Verification items for the finished model (mm, model axes). A direction names the side the tool comes from. Round coordinates to 2 decimals unless told otherwise and drop trailing zeros. Write each loop counter-clockwise with the first axis right and the second up, starting at its lowest first coordinate (ties: lowest second). Pieces come first, ordered by that corner, then holes. Notation, with made-up numbers: (59, -20) -> (111, -20) arc R4 ccw to (111, -16) -> close; hole circle Ø2 at (66, -38). An arc over 180 degrees is marked (long way). Use CSV: the item, a comma, the result in double quotes.
```python
from build123d import *

# Parameters (mm, degrees)
BOSS_EXTRUDE1_DEPTH                                = 304.8
SKETCH2_R                                          = 2.3876
CUT_EXTRUDE1_DEPTH                                 = 317.354227758
SKETCH3_R                                          = 11.1125
CUT_EXTRUDE2_DEPTH                                 = 304.8
CSK_FOR_10_FLAT_HEAD_MACHINE_SCREW1_AT_COUNT       = 2
CSK_FOR_10_FLAT_HEAD_MACHINE_SCREW1_AT_PITCH       = 41.275
LPATTERN1_COUNT                                    = 2
LPATTERN1_PITCH                                    = 171.958
FILLET1_R                                          = 6.35
SKETCH14_R                                         = 4.8895
SKETCH14_R_2                                       = 2.8067
BOSS_EXTRUDE2_DEPTH                                = 3.175
CONVERT_SOLID1_DEPTH                               = 304.8
F_10_0_1935_DIAMETER_HOLE1_D                       = 4.9149
F_10_0_1935_DIAMETER_HOLE1_DEPTH                   = 3.048
CSK_FOR_10_FLAT_HEAD_MACHINE_SCREW_100_D           = 5.6134
CSK_FOR_10_FLAT_HEAD_MACHINE_SCREW_100_DEPTH       = 36.8935
CSK_FOR_10_FLAT_HEAD_MACHINE_SCREW_100_CSINK_D     = 9.779
CSK_FOR_10_FLAT_HEAD_MACHINE_SCREW_100_CSINK_ANGLE = 82


# Read off the part's stored shape, not the designer's step: Convert-Solid1
with BuildPart() as part:
    # Sketch1 → Boss-Extrude1 (new body)
    with BuildSketch(Plane(origin=(0, 0, 0), x_dir=(0, 0, -1), z_dir=(1, 0, 0))):
        with BuildLine():
            Line((-76.2, 4.2545), (-53.975, 4.2545))
            ThreePointArc((-53.975, 4.2545), (-49.484871939, 6.114371939), (-47.625, 10.6045))
            Line((-47.625, 10.6045), (-47.625, 34.925))
            ThreePointArc((-47.625, 34.925), (-46.69506403, 37.17006403), (-44.45, 38.1))
            Line((-44.45, 38.1), (44.45, 38.1))
            ThreePointArc((44.45, 38.1), (46.69506403, 37.17006403), (47.625, 34.925))
            Line((47.625, 34.925), (47.625, 10.6045))
            ThreePointArc((47.625, 10.6045), (49.484871939, 6.114371939), (53.975, 4.2545))
            Line((53.975, 4.2545), (76.2, 4.2545))
            Line((76.2, 4.2545), (76.2, 7.4295))
            Line((76.2, 7.4295), (53.975, 7.4295))
            ThreePointArc((53.975, 7.4295), (51.72993597, 8.35943597), (50.8, 10.6045))
            Line((50.8, 10.6045), (50.8, 34.925))
            ThreePointArc((50.8, 34.925), (48.940128061, 39.415128061), (44.45, 41.275))
            Line((44.45, 41.275), (-44.45, 41.275))
            ThreePointArc((-44.45, 41.275), (-48.940128061, 39.415128061), (-50.8, 34.925))
            Line((-50.8, 34.925), (-50.8, 10.6045))
            ThreePointArc((-50.8, 10.6045), (-51.72993597, 8.35943597), (-53.975, 7.4295))
            Line((-53.975, 7.4295), (-76.2, 7.4295))
            Line((-76.2, 7.4295), (-76.2, 4.2545))
        make_face()
    extrude(amount=BOSS_EXTRUDE1_DEPTH)

    # Sketch2 → Cut-Extrude1 (cut, through all)
    with BuildSketch(Plane.XZ.offset(-4.2545)):
        with Locations(Location((25.4, 63.5, 0), (0, 0, 270))):
            Circle(SKETCH2_R)
        with Locations(Location((152.4, 63.5, 0), (0, 0, 270))):
            Circle(SKETCH2_R)
        with Locations(Location((279.4, 63.5, 0), (0, 0, 270))):
            Circle(SKETCH2_R)
    cut_extrude1 = extrude(amount=-CUT_EXTRUDE1_DEPTH, mode=Mode.SUBTRACT)

    # Mirror1: Cut-Extrude1 across plane
    add(cut_extrude1.mirror(Plane.XY), mode=Mode.SUBTRACT)

    # Sketch3 → Cut-Extrude2 (cut)
    with BuildSketch(Plane(origin=(0, 41.275, 0), x_dir=(1, 0, 0), z_dir=(0, 1, 0))):
        with Locations(Location((66.675, -15.875, 0), (0, 0, 270))):
            Circle(SKETCH3_R)
    cut_extrude2 = extrude(amount=-CUT_EXTRUDE2_DEPTH, mode=Mode.SUBTRACT)

    # Sketch5 → CSK for #10 Flat Head Machine Screw1 (revolve, cut)
    with BuildSketch(Plane(origin=(46.0375, 41.275, 15.875), x_dir=(0, 0, 1), z_dir=(1, 0, 0))):
        Polygon((0, 0), (0, 3.175), (2.8067, 3.175), (2.8067, 2.395987319), (4.8895, 0), align=None)
    csk_for_10_flat_head_machine_screw1 = revolve(axis=Axis((46.0375, 47.625, 15.875), (0, -1, 0)), mode=Mode.SUBTRACT)

    # CSK for #10 Flat Head Machine Screw1 at: CSK for #10 Flat Head Machine Screw1 ×2
    with Locations(*[(i * CSK_FOR_10_FLAT_HEAD_MACHINE_SCREW1_AT_PITCH, 0, 0) for i in range(1, CSK_FOR_10_FLAT_HEAD_MACHINE_SCREW1_AT_COUNT)]):
        add(csk_for_10_flat_head_machine_screw1, mode=Mode.SUBTRACT)

    # LPattern1: Cut-Extrude2, CSK for #10 Flat Head Machine Screw1 ×2
    with Locations(*[(i * LPATTERN1_PITCH, 0, 0) for i in range(1, LPATTERN1_COUNT)]):
        add(cut_extrude2, mode=Mode.SUBTRACT)
        add(csk_for_10_flat_head_machine_screw1, mode=Mode.SUBTRACT)

    # LPattern1 copy 1 sketch → LPattern1 copy 1 (revolve, cut)
    with BuildSketch(Plane(origin=(259.2705, 41.275, 15.875), x_dir=(0, 0, 1), z_dir=(1, 0, 0))):
        Polygon((0, 0), (0, 3.175), (2.8067, 3.175), (2.8067, 2.395987319), (4.8895, 0), align=None)
    revolve(axis=Axis((259.2705, 47.625, 15.875), (0, -1, 0)), mode=Mode.SUBTRACT)

    # Fillet1
    fillet1_edges = [part.edges().sort_by_distance(p)[0] for p in [
        (0, 5.842, -76.2),
        (0, 5.842, 76.2),
        (304.8, 5.842, -76.2),
        (304.8, 5.842, 76.2),
    ]]
    fillet(fillet1_edges, radius=FILLET1_R)

    # Sketch14 → Boss-Extrude2 (add)
    # profile 1 of 4: a face of its own
    with BuildSketch(Plane(origin=(0, 41.275, 0), x_dir=(1, 0, 0), z_dir=(0, 1, 0))):
        with Locations((259.2705, -15.875)):
            Circle(SKETCH14_R)
        with Locations(Location((259.2705, -15.875, 0), (0, 0, 270))):
            Circle(SKETCH14_R_2, mode=Mode.SUBTRACT)
    # profile 2 of 4: a face of its own
    with BuildSketch(Plane(origin=(0, 41.275, 0), x_dir=(1, 0, 0), z_dir=(0, 1, 0))):
        with Locations((87.3125, -15.875)):
            Circle(SKETCH14_R)
        with Locations(Location((87.3125, -15.875, 0), (0, 0, 270))):
            Circle(SKETCH14_R_2, mode=Mode.SUBTRACT)
    # profile 3 of 4: a face of its own
    with BuildSketch(Plane(origin=(0, 41.275, 0), x_dir=(1, 0, 0), z_dir=(0, 1, 0))):
        with Locations((217.9955, -15.875)):
            Circle(SKETCH14_R)
        with Locations(Location((217.9955, -15.875, 0), (0, 0, 270))):
            Circle(SKETCH14_R_2, mode=Mode.SUBTRACT)
    # profile 4 of 4: a face of its own
    with BuildSketch(Plane(origin=(0, 41.275, 0), x_dir=(1, 0, 0), z_dir=(0, 1, 0))):
        with Locations((46.0375, -15.875)):
            Circle(SKETCH14_R)
        with Locations(Location((46.0375, -15.875, 0), (0, 0, 270))):
            Circle(SKETCH14_R_2, mode=Mode.SUBTRACT)
    extrude(amount=-BOSS_EXTRUDE2_DEPTH)

    # Convert-Solid1 outline → Convert-Solid1 (cut)
    with BuildSketch(Plane.YZ):
        with BuildLine():
            Line((4.3815, -76.2), (4.3815, -53.975))
            ThreePointArc((4.3815, -53.975), (6.204174501, -49.574674501), (10.6045, -47.752))
            Line((10.6045, -47.752), (34.925, -47.752))
            ThreePointArc((34.925, -47.752), (37.259866591, -46.784866591), (38.227, -44.45))
            Line((38.227, -44.45), (38.227, 44.45))
            ThreePointArc((38.227, 44.45), (37.259866591, 46.784866591), (34.925, 47.752))
            Line((34.925, 47.752), (10.6045, 47.752))
            ThreePointArc((10.6045, 47.752), (6.204174501, 49.574674501), (4.3815, 53.975))
            Line((4.3815, 53.975), (4.3815, 76.2))
            Line((4.3815, 76.2), (4.2545, 76.2))
            Line((4.2545, 76.2), (4.2545, 53.975))
            ThreePointArc((4.2545, 53.975), (6.114371939, 49.484871939), (10.6045, 47.625))
            Line((10.6045, 47.625), (34.925, 47.625))
            ThreePointArc((34.925, 47.625), (37.17006403, 46.69506403), (38.1, 44.45))
            Line((38.1, 44.45), (38.1, -44.45))
            ThreePointArc((38.1, -44.45), (37.17006403, -46.69506403), (34.925, -47.625))
            Line((34.925, -47.625), (10.6045, -47.625))
            ThreePointArc((10.6045, -47.625), (6.114371939, -49.484871939), (4.2545, -53.975))
            Line((4.2545, -53.975), (4.2545, -76.2))
            Line((4.2545, -76.2), (4.3815, -76.2))
        make_face()
    extrude(amount=CONVERT_SOLID1_DEPTH, mode=Mode.SUBTRACT)

    # #10 (0.1935) Diameter Hole1
    with Locations(Plane(origin=(0, 7.4295, 0), x_dir=(1, 0, 0), z_dir=(0, 1, 0))):
        with Locations((25.4, 63.5), (152.4, 63.5), (279.4, 63.5), (279.4, -63.5), (152.4, -63.5), (25.4, -63.5)):
            Hole(F_10_0_1935_DIAMETER_HOLE1_D / 2, depth=F_10_0_1935_DIAMETER_HOLE1_DEPTH)

    # CSK for #10 Flat Head Machine Screw (100)1
    with Locations(Plane(origin=(0, 41.275, 0), x_dir=(1, 0, 0), z_dir=(0, 1, 0))):
        with Locations((46.0375, -15.875), (87.3125, -15.875), (217.9955, -15.875), (259.2705, -15.875)):
            CounterSinkHole(CSK_FOR_10_FLAT_HEAD_MACHINE_SCREW_100_D / 2, CSK_FOR_10_FLAT_HEAD_MACHINE_SCREW_100_CSINK_D / 2, depth=CSK_FOR_10_FLAT_HEAD_MACHINE_SCREW_100_DEPTH, counter_sink_angle=CSK_FOR_10_FLAT_HEAD_MACHINE_SCREW_100_CSINK_ANGLE)


solid = part.part
```
Q1. Mould release check, pull along X, two halves, no side actions. Record for faces 5 (the cylindrical face through (1.91, 5.88, 74.39)), 6 (the cylindrical face through (150.27, 6.25, 49.53)), 7 (the conical face through (256.58, 39, 16.99)), 8 (the cylindrical face through (302.99, 5.93, -74.29)): released by +X, released by -X, zero draft, split by the parting line, or undercut.
Filled in:
face 5,"released by -X"
face 6,"zero draft"
face 7,"undercut"
face 8,"released by +X"
Q2. Section check C-C (z = -19). Record the cut outline in (x, y) (3 decimals).
Filled in:
outline,"(0, 38.227) -> (304.8, 38.227) -> (304.8, 41.275) -> (0, 41.275) -> close"
Q3. Section check A-A (y = 26.5). Record the cut outline in (x, z).
Filled in:
outline,"(0, -50.8) -> (304.8, -50.8) -> (304.8, -47.75) -> (0, -47.75) -> close; (0, 47.75) -> (304.8, 47.75) -> (304.8, 50.8) -> (0, 50.8) -> close"
Q4. Access from +Z, -Z, +X, -X, +Y, -Y to the whole of each face (thin tool, end or side, straight path). Record for faces 1 (the flat face through (150, 23, -50.8)), 2 (the flat face through (150, 23, 50.8)), 3 (the flat face through (150, 23, 47.752)), 4 (the cylindrical face through (220.735, 38.558, 15.267)).
Filled in:
face 1,"-Z, +X, -X, +Y"
face 2,"+Z, +X, -X, +Y"
face 3,"+X, -X, -Y"
face 4,"+Y, -Y"
Q5. Material ranges on L1, parallel to X at y = 5.95, z = 63.5; L2, parallel to Z at x = 238.5, y = 26; L3, parallel to X at y = 6, z = -63, recorded low to high.
Filled in:
L1,"0 to 22.94, 27.86 to 149.94, 154.86 to 276.94, 281.86 to 304.8"
L2,"-50.8 to -47.75, 47.75 to 50.8"
L3,"0 to 22.99, 27.81 to 149.99, 154.81 to 276.99, 281.81 to 304.8"
Q6. Go/stop test with flat-tipped pins: P1, Ø9, axis at x = 46.04, z = 15.88, coming from the -Y side; P2, Ø11, axis at x = 163, z = 61, coming from the +Y side; P3, Ø10, axis at x = 139, y = 21.5, coming from the -Z side. Record where each tip stops, or that it passes through.
Filled in:
P1,"y = 38.23"
P2,"y = 7.43"
P3,"z = -50.8"
